```python
from build123d import *

# Parameters (mm, degrees)
SKETCH1_W           = 25.4
SKETCH1_H           = 25.4
BOSS_EXTRUDE1_DEPTH = 177.8
FILLET1_R           = 1.5875
HOLE1_OUTLINE_R     = 2.5527
HOLE1_DEPTH         = 177.8
SKETCH7_W           = 6.5278
SKETCH7_H           = 2.2352
CUT_EXTRUDE2_DEPTH  = 177.8
FILLET4_R           = 0.396875
CIRPATTERN2_DEPTH   = 177.8
CUT_EXTRUDE3_DEPTH  = 181.05357536


# Read off the part's stored shape, not the designer's step: Hole1, CirPattern2
with BuildPart() as part:
    # Sketch1 → Boss-Extrude1 (new body)
    with BuildSketch(Plane.XY):
        Rectangle(SKETCH1_W, SKETCH1_H)
    extrude(amount=BOSS_EXTRUDE1_DEPTH)

    # Fillet1
    fillet1_edges = [part.edges().sort_by_distance(p)[0] for p in [
        (12.7, -12.7, 88.9),
        (-12.7, -12.7, 88.9),
        (-12.7, 12.7, 88.9),
        (12.7, 12.7, 88.9),
    ]]
    fillet(fillet1_edges, radius=FILLET1_R)

    # Hole1 outline → Hole1 (cut)
    with BuildSketch(Plane.XY):
        with Locations((0, -0.048792482)):
            Circle(HOLE1_OUTLINE_R)
    extrude(amount=HOLE1_DEPTH, mode=Mode.SUBTRACT)

    # Sketch7 → Cut-Extrude2 (cut)
    with BuildSketch(Plane.XY.offset(177.8)):
        with Locations((0, 11.5824)):
            Rectangle(SKETCH7_W, SKETCH7_H)
        Polygon((-3.175, 4.5212), (-7.3025, 10.4648), (7.3025, 10.4648), (3.175, 4.5212), align=None)
    extrude(amount=-CUT_EXTRUDE2_DEPTH, mode=Mode.SUBTRACT)

    # Fillet4
    fillet4_edges = [part.edges().sort_by_distance(p)[0] for p in [
        (-3.2639, 10.4648, 88.9),
        (-3.2639, 12.7, 88.9),
        (3.2639, 12.7, 88.9),
        (3.2639, 10.4648, 88.9),
    ]]
    fillet(fillet4_edges, radius=FILLET4_R)

    # CirPattern2 outline → CirPattern2 (cut)
    with BuildSketch(Plane.XY):
        with BuildLine():
            ThreePointArc((-3.660775, -10.562384964), (-3.380141996, -10.67862696), (-3.2639, -10.959259964))
            Line((-3.2639, -10.959259964), (-3.2639, -12.7))
            Line((-3.2639, -12.7), (3.2639, -12.7))
            Line((3.2639, -12.7), (3.2639, -10.959259964))
            ThreePointArc((3.2639, -10.959259964), (3.380141996, -10.67862696), (3.660775, -10.562384964))
            Line((3.660775, -10.562384964), (7.3025, -10.562384964))
            Line((7.3025, -10.562384964), (3.175, -4.618784964))
            Line((3.175, -4.618784964), (-3.175, -4.618784964))
            Line((-3.175, -4.618784964), (-7.3025, -10.562384964))
            Line((-7.3025, -10.562384964), (-3.660775, -10.562384964))
        make_face()
        with BuildLine():
            Line((-12.7, -3.312692482), (-10.910467482, -3.312692482))
            ThreePointArc((-10.910467482, -3.312692482), (-10.629834478, -3.428934478), (-10.513592482, -3.709567482))
            Line((-10.513592482, -3.709567482), (-10.513592482, -7.351292482))
            Line((-10.513592482, -7.351292482), (-4.569992482, -3.223792482))
            Line((-4.569992482, -3.223792482), (-4.569992482, 3.126207518))
            Line((-4.569992482, 3.126207518), (-10.513592482, 7.253707518))
            Line((-10.513592482, 7.253707518), (-10.513592482, 3.611982518))
            ThreePointArc((-10.513592482, 3.611982518), (-10.629834478, 3.331349514), (-10.910467482, 3.215107518))
            Line((-10.910467482, 3.215107518), (-12.7, 3.215107518))
            Line((-12.7, 3.215107518), (-12.7, -3.312692482))
        make_face()
        with BuildLine():
            ThreePointArc((10.513592482, -3.709567482), (10.629834478, -3.428934478), (10.910467482, -3.312692482))
            Line((10.910467482, -3.312692482), (12.7, -3.312692482))
            Line((12.7, -3.312692482), (12.7, 3.215107518))
            Line((12.7, 3.215107518), (10.910467482, 3.215107518))
            ThreePointArc((10.910467482, 3.215107518), (10.629834478, 3.331349514), (10.513592482, 3.611982518))
            Line((10.513592482, 3.611982518), (10.513592482, 7.253707518))
            Line((10.513592482, 7.253707518), (4.569992482, 3.126207518))
            Line((4.569992482, 3.126207518), (4.569992482, -3.223792482))
            Line((4.569992482, -3.223792482), (10.513592482, -7.351292482))
            Line((10.513592482, -7.351292482), (10.513592482, -3.709567482))
        make_face()
    extrude(amount=CIRPATTERN2_DEPTH, mode=Mode.SUBTRACT)

    # Sketch8 → Cut-Extrude3 (cut, through all)
    with BuildSketch(Plane(origin=(12.7, 0, 0), x_dir=(0, 0, -1), z_dir=(1, 0, 0))):
        Polygon((0, 12.7), (0, -12.7), (-6.191852564, 12.7), align=None)
    extrude(amount=-CUT_EXTRUDE3_DEPTH, mode=Mode.SUBTRACT)


solid = part.part
```
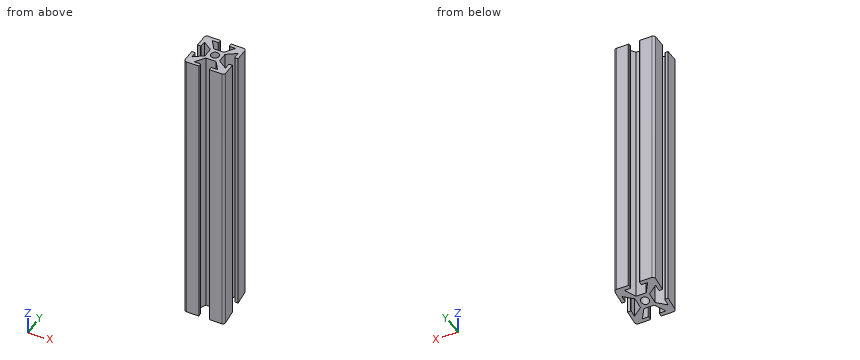
Input: part model. Units: mm. Frame: model coordinates. Round coordinates to 2 decimals unless told otherwise and drop trailing zeros. Loops run counter-clockwise (first coordinate to the right, second up) from the corner with the lowest first, then second, coordinate; pieces in that order, holes last. Notation, with made-up numbers: (-5.75, 29.5) - (12.25, 29.5) arc R15 ccw to (12.25, 40.5) - close; hole circle Ø11 at (30, 16). An arc over 180 degrees is marked (long way). One line per item, written item: value. Start each with the question number.
(1) Ray query, line 1 (Y direction, x = 0, z = 64); line 2 (X direction, y = -6.5, z = 64); line 3 (X direction, y = 0.25, z = 127). Return the intervals inside material, ascending. Write a range as [from, to].
(2) Section A-A, the plane x = 0. Return loops of the section in (y, z).
(3) Contact query for flat-ended pins moving along their axis: P1, Ø0.9, axis at x = 12, z = 102.5, coming from the +Y side; P2, Ø1.5, axis at x = 9.5, y = -1.5, coming from the +Z side; P3, Ø1.9, axis at x = -1, z = 81.5, coming from the -Y side; P4, Ø1, axis at y = -1, z = 156, coming from the -X side. Output: stop coordinate, or through.
Results below:
1. line 1: [-4.62, -2.6], [2.5, 4.52]
1. line 2: [-12.7, -10.51], [-9.29, -4.48], [4.48, 9.29], [10.51, 12.7]
1. line 3: [-4.57, -2.54], [2.54, 4.57]
2. outline: (-4.62, 1.97) - (-2.6, 2.46) - (-2.6, 177.8) - (-4.62, 177.8) - close; (2.5, 3.71) - (4.52, 4.2) - (4.52, 177.8) - (2.5, 177.8) - close
3. P1: y = 12.64
3. P2: through
3. P3: y = -4.62
3. P4: x = -4.57
